The model under review builds one solid part; all positions refer to its coordinate system, in mm. Face numbers are marked on the shaded views. A direction names the side the tool comes from. Give positions to 0.01 mm unless a question says otherwise; leave off trailing zeros. Write each loop counter-clockwise with the first axis right and the second up, starting at its lowest first coordinate (ties: lowest second). Pieces come first, ordered by that corner, then holes. Notation, with made-up numbers: M -32,23.25 L -3,23.25 A27 cw -3,48.25 Z; hole C -26.5,-10 d4. An arc over 180 degrees is marked long. Write each question's results on one line, items separated by ' | '. Start each with the question number.
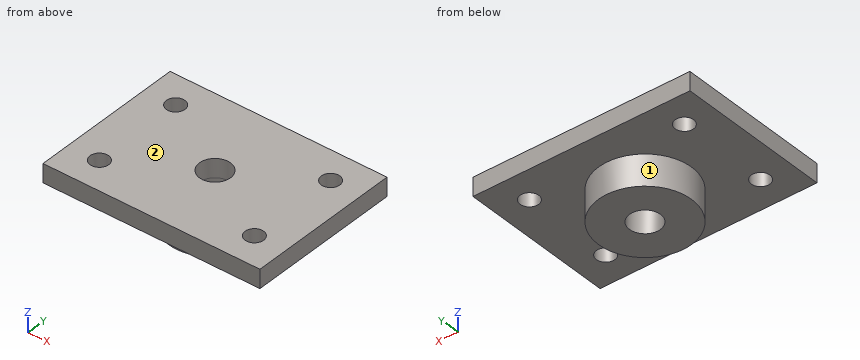
from build123d import *

# Parameters (mm, degrees)
SKETCH1_W           = 35
SKETCH1_H           = 25
BOSS_EXTRUDE1_DEPTH = 3
SKETCH2_R           = 2.5
SKETCH2_R_2         = 1.5
CUT_EXTRUDE1_DEPTH  = 3
SKETCH3_R           = 7.5
SKETCH3_R_2         = 2.5
BOSS_EXTRUDE2_DEPTH = 5


with BuildPart() as part:
    # Sketch1 → Boss-Extrude1 (new body)
    with BuildSketch(Plane.XY):
        Rectangle(SKETCH1_W, SKETCH1_H)
    extrude(amount=BOSS_EXTRUDE1_DEPTH)

    # Sketch2 → Cut-Extrude1 (cut)
    with BuildSketch(Plane.XY.offset(3)):
        Circle(SKETCH2_R)
        with Locations((-12.5, 7.5)):
            Circle(SKETCH2_R_2)
        with Locations((12.5, 7.5)):
            Circle(SKETCH2_R_2)
        with Locations((12.5, -7.5)):
            Circle(SKETCH2_R_2)
        with Locations((-12.5, -7.5)):
            Circle(SKETCH2_R_2)
    extrude(amount=-CUT_EXTRUDE1_DEPTH, mode=Mode.SUBTRACT)

    # Sketch3 → Boss-Extrude2 (add)
    with BuildSketch(Plane(origin=(0, 0, 0), x_dir=(-1, 0, 0), z_dir=(0, 0, -1))):
        with Locations(Location((0, 0, 0), (0, 0, 180))):
            Circle(SKETCH3_R)
        with Locations(Location((0, 0, 0), (0, 0, 180))):
            Circle(SKETCH3_R_2, mode=Mode.SUBTRACT)
    extrude(amount=BOSS_EXTRUDE2_DEPTH)


solid = part.part
(1) Wall thickness on L1, parallel to Y at x = 12.5, z = 2.3; L2, parallel to X at y = -7, z = 1; L3, parallel to Z at x = -15, y = 2.25: over which ranges is each line inside the solid? List them lowest first.
(2) Clearance check with flat-ended pins moving along their axes: P1, Ø3, axis at x = 0, y = 0, coming from the +Z side; P2, Ø3.5, axis at x = 12.5, y = 7.5, coming from the +Z side; P3, Ø1.5, axis at y = -3.5, z = -2.5, coming from the -X side; P4, Ø2, axis at x = -10.5, y = 2, coming from the -Z side. State where each tip first meets the part, or that it passes through.
(3) Machinability: for the marked faces 1 and 2, which of the approach directions +Z, -Z, +X, -X, +Y, -Y give a long, thin tool a straight path to every point of the face, cutting with its end or side? Answer none if there is none.
(4) Add section D-D (z = -1). State the section outline as (x, y) points.
(5) Add section C-C (x = 12.5). State the section outline as (y, z) points.
(6) Add section A-A (x = 0). State the section outline as (y, z) points.
(7) Add section B-B (y = 0). State the section outline as (x, z) points.
Calculated:
1) L1: y = -12.5 to -9, -6 to 6, 9 to 12.5 | L2: x = -17.5 to -13.91, -11.09 to 11.09, 13.91 to 17.5 | L3: z = 0 to 3
2) P1: passes through | P2: stops at z = 3 | P3: stops at x = -6.98 | P4: stops at z = 0
3) face 1: -Z | face 2: +Z, +X, -X, +Y, -Y
4) outline: C 0,0 d15; hole C 0,0 d5
5) outline: M -12.5,0 L -9,0 L -9,3 L -12.5,3 Z; M -6,0 L 6,0 L 6,3 L -6,3 Z; M 9,0 L 12.5,0 L 12.5,3 L 9,3 Z
6) outline: M -12.5,0 L -7.5,0 L -7.5,-5 L -2.5,-5 L -2.5,3 L -12.5,3 Z; M 2.5,-5 L 7.5,-5 L 7.5,0 L 12.5,0 L 12.5,3 L 2.5,3 Z
7) outline: M -17.5,0 L -7.5,0 L -7.5,-5 L -2.5,-5 L -2.5,3 L -17.5,3 Z; M 2.5,-5 L 7.5,-5 L 7.5,0 L 17.5,0 L 17.5,3 L 2.5,3 Z
